CAD build for the part. Positions are in the model's coordinates, mm. Face numbers are marked on the shaded views. Coordinates: 2 decimals unless noted, no trailing zeros. Write each loop counter-clockwise with the first axis right and the second up, starting at its lowest first coordinate (ties: lowest second). Pieces come first, ordered by that corner, then holes. Notation, with made-up numbers: (26.5, -28.75) -> (63.5, -28.75) arc R19 ccw to (63.5, 8.25) -> close; hole circle Ø6 at (42, 38.25). An arc over 180 degrees is marked (long way). Answer as CSV lines item,"result".
Autodesk Inventor part; units mm, degrees
ref_plane "YZ Plane" through (0, 0, 0) normal (1, 0, 0) x (0, 1, 0)
ref_plane "XZ Plane" through (0, 0, 0) normal (0, 1, 0) x (-1, 0, 0)
ref_plane "XY Plane" through (0, 0, 0) normal (0, 0, 1) x (1, 0, 0)
sketch "スケッチ1" plane through (0, 0, 0) normal (0, 0, 1) x (1, 0, 0)
  line L0 (0, 20) -> (100, 20)
  line L1 (100, 20) -> (100, -20)
  line L2 (100, -20) -> (0, -20)
  line L3 (0, -20) -> (0, 20)
  circle A0 centre (0, 0) radius 20
  dimension "d0" = 100
  dimension "d1" = 40
  dimension "d2" = 20
  dimension "d3" = 100
extrude "押し出し1" add sketch "スケッチ1" along normal mid plane 20
sketch "スケッチ2" plane through (0, 0, 10) normal (0, 0, 1) x (1, 0, 0)
  circle A0 centre (0, 0) radius 5
  dimension "d6" = 10
extrude "押し出し2" cut sketch "スケッチ2" against normal through all
equation "\"d7\" = d6"
properties part number "Base" material "ゴールド"
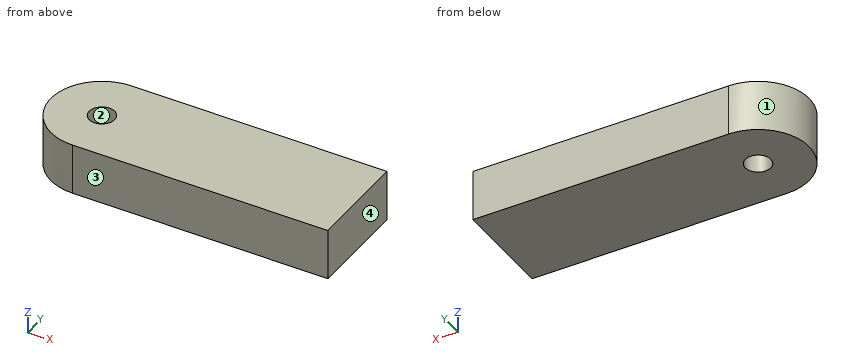
Item 1: Wall check: line 1 (Y direction, x = 0, z = 3.75); line 2 (X direction, y = -0.5, z = 8); line 3 (Y direction, x = -1.5, z = -3.5). Give the ranges that are in metal, low to high. Write a range as from..to.
Answer below:
line 1,"y = -20..-5, 5..20"
line 2,"x = -19.99..-4.97, 4.97..100"
line 3,"y = -19.94..-4.77, 4.77..19.94"
Item 2: Saw through at D-D on y = -12. Give the cut face in (x, z), and give its area (3 significant figures).
Answer below:
outline,"(-16, -10) -> (100, -10) -> (100, 10) -> (-16, 10) -> close"
area,"2,320 mm2"
Item 3: Saw through at B-B on z = 8. Give the cut face in (x, y), and give its area (3 significant figures).
Answer below:
outline,"(0, -20) -> (100, -20) -> (100, 20) -> (0, 20) arc R20 ccw to start; hole circle Ø10 at (0, 0)"
area,"4,550 mm2"
Item 4: Two-plate mould, pull along Y, no slides. Class the marked faces 1, 2, 3 and 4: pulls with the +Y half, pulls with the -Y half, needs draft (parallel to the pull), parting line crosses it, or undercut.
Answer below:
face 1,"parting line crosses it"
face 2,"undercut"
face 3,"pulls with the -Y half"
face 4,"needs draft"
Item 5: Saw through at C-C on x = -1.5. Give the cut face in (y, z), and give its area (3 significant figures).
Answer below:
outline,"(-19.94, -10) -> (-4.77, -10) -> (-4.77, 10) -> (-19.94, 10) -> close; (4.77, -10) -> (19.94, -10) -> (19.94, 10) -> (4.77, 10) -> close"
area,"607 mm2"
Item 6: Flat gauge pins, fed straight in: pin 1 (11.5 mm diameter, centred on x = 0, y = 0, fed in from -Z); pin 2 (3 mm diameter, centred on y = -14.5, z = -4, fed in from -X); pin 3 (8 mm diameter, centred on y = -3, z = 6, fed in from -X). Where does each tip first touch, or does it go through?
Answer below:
pin 1,"stops at z = -10"
pin 2,"stops at x = -15.2"
pin 3,"stops at x = -20"
Item 7: Saw through at A-A on y = 0. Give the cut face in (x, z), and give its area (3 significant figures).
Answer below:
outline,"(-20, -10) -> (-5, -10) -> (-5, 10) -> (-20, 10) -> close; (5, -10) -> (100, -10) -> (100, 10) -> (5, 10) -> close"
area,"2,200 mm2"
